Answer from the drawing. Dimensions are ordinates in mm from the lowest x, y and z of the part. Round coordinates to 2 decimals unless told otherwise and drop trailing zeros. Loops run counter-clockwise (first coordinate to the right, second up) from the corner with the lowest first, then second, coordinate; pieces in that order, holes last.
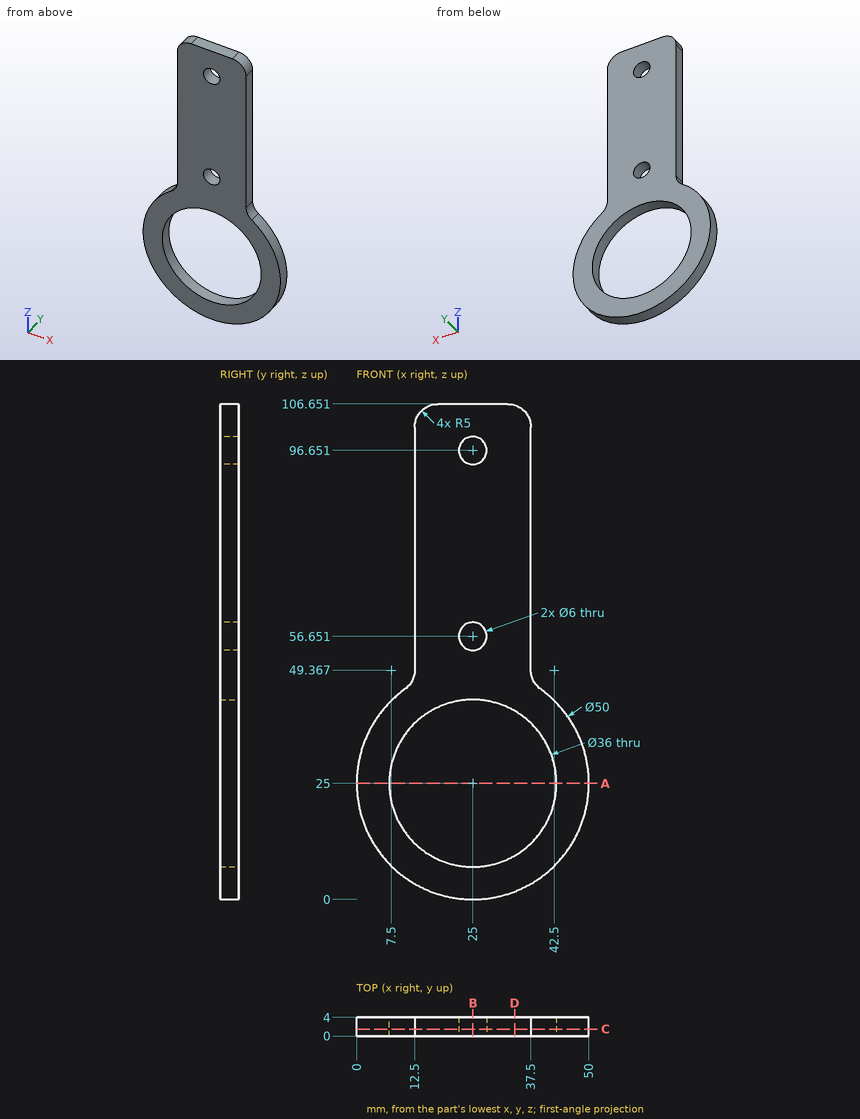
1. Find section D-D (x = 34). Write down the section's boundary in (y, z), then the cut area to 3 significant figures.
Answer key:
outline: (0, 1.68) - (4, 1.68) - (4, 9.41) - (0, 9.41) - close; (0, 40.59) - (4, 40.59) - (4, 106.42) - (0, 106.42) - close
area: 294 mm2
2. Find section B-B (x = 25). Write down the section's boundary in (y, z).
Answer key:
outline: (0, 0) - (4, 0) - (4, 7) - (0, 7) - close; (0, 43) - (4, 43) - (4, 53.65) - (0, 53.65) - close; (0, 59.65) - (4, 59.65) - (4, 93.65) - (0, 93.65) - close; (0, 99.65) - (4, 99.65) - (4, 106.65) - (0, 106.65) - close
3. Given pin 1 (1 mm diameter, centred on y = 2.5, z = 11, fed in from +X); pin 2 (10 mm diameter, centred on x = 16, z = 29, fed in from -Y); pin 3 (2 mm diameter, centred on y = 2.5, z = 80, fed in from +X); pin 4 (9.5 mm diameter, centred on x = 25, z = 96.65, fed in from -Y), each flat-ended and moving along its own axis, determine where each tip first touches the part or whether it passes through.
Answer key:
pin 1: stops at x = 46.04
pin 2: passes through
pin 3: stops at x = 37.5
pin 4: stops at y = 0
4. Consider probe 1 along Z at (x, y) = (25, 2.7); probe 2 along X at (y, z) = (3.55, 68.5); probe 3 along Z at (x, y) = (37, 2.15) (1 decimal). Determine where each line is inside the solid, lowest interval first.
Answer key:
probe 1: z = 0 to 7, 43 to 53.65, 59.65 to 93.65, 99.65 to 106.65
probe 2: x = 12.5 to 37.5
probe 3: z = 3.1 to 11.6, 38.4 to 103.8
5. Find section C-C (y = 1.5). Write down the section's boundary in (x, z), then the cut area to 3 significant figures.
Answer key:
outline: (10.42, 45.31) arc R25 ccw (long way) to (39.58, 45.31) arc R5 cw to (37.5, 49.37) - (37.5, 101.65) arc R5 ccw to (32.5, 106.65) - (17.5, 106.65) arc R5 ccw to (12.5, 101.65) - (12.5, 49.37) arc R5 cw to start; hole circle Ø36 at (25, 25); hole circle Ø6 at (25, 56.65); hole circle Ø6 at (25, 96.65)
area: 2,320 mm2
6. Find section A-A (z = 25). Write down the section's boundary in (x, y), then the cut area to 3 significant figures.
Answer key:
outline: (0, 0) - (7, 0) - (7, 4) - (0, 4) - close; (43, 0) - (50, 0) - (50, 4) - (43, 4) - close
area: 56.0 mm2
